from build123d import *

# Parameters (mm, degrees)
SKETCH_3_W          = 88.5
SKETCH_3_H          = 114.5
SKETCH_3_W_2        = 36.5
SKETCH_3_H_2        = 36.5
SKETCH_3_W_3        = 50.5
SKETCH_3_H_3        = 73.5
SKETCH_3_W_4        = 33.5
SKETCH_3_H_4        = 70.5
SKETCH_3_W_5        = 25.5
SKETCH_3_H_5        = 21.5
EXTRUDE_1_DEPTH     = 25
SKETCH_3_3_W        = 36.5
SKETCH_3_3_H        = 36.5
SKETCH_3_3_R        = 2.1
SKETCH_3_3_W_2      = 50.5
SKETCH_3_3_H_2      = 73.5
SKETCH_3_3_W_3      = 33.5
SKETCH_3_3_H_3      = 70.5
SKETCH_3_3_R_2      = 2.5
SKETCH_3_3_W_4      = 25.5
SKETCH_3_3_H_4      = 21.5
EXTRUDE_2_DEPTH     = 1.5
SKETCH_3_5_R        = 2.1
SKETCH_3_5_R_2      = 1.25
SKETCH_3_5_R_3      = 2.5
SKETCH_3_5_R_4      = 1.5
EXTRUDE_4_DEPTH     = 4.5
CUT_EXTRUDE_1_DEPTH = 17.5
CUT_EXTRUDE_2_REACH = 148.859
SKETCH_5_W          = 40
SKETCH_5_H          = 10
SKETCH_5_W_2        = 11
SKETCH_5_H_2        = 5


with BuildPart() as part:
    # 草图3 → 凸台-拉伸1 (new body)
    with BuildSketch(Plane(origin=(0, 0, 0), x_dir=(1, 0, 0), z_dir=(0, 1, 0))):
        with Locations((44.25, 57.25)):
            Rectangle(SKETCH_3_W, SKETCH_3_H)
        Polygon((39.5, 1.5), (39.5, 38), (53.5, 38), (53.5, 41), (87, 41), (87, 24.5), (60, 24.5), (60, 1.5), align=None, mode=Mode.SUBTRACT)
        with Locations((19.75, 19.75)):
            Rectangle(SKETCH_3_W_2, SKETCH_3_H_2, mode=Mode.SUBTRACT)
        with Locations((26.75, 76.25)):
            Rectangle(SKETCH_3_W_3, SKETCH_3_H_3, mode=Mode.SUBTRACT)
        with Locations((70.25, 77.75)):
            Rectangle(SKETCH_3_W_4, SKETCH_3_H_4, mode=Mode.SUBTRACT)
        with Locations((74.25, 12.25)):
            Rectangle(SKETCH_3_W_5, SKETCH_3_H_5, mode=Mode.SUBTRACT)
    extrude(amount=EXTRUDE_1_DEPTH)

    # 草图3<3> → 凸台-拉伸2 (add)
    # profile 1 of 5: a face of its own
    with BuildSketch(Plane(origin=(0, 0, 0), x_dir=(1, 0, 0), z_dir=(0, 1, 0))):
        Polygon((39.5, 38), (39.5, 1.5), (60, 1.5), (60, 24.5), (87, 24.5), (87, 41), (53.5, 41), (53.5, 38), align=None)
    # profile 2 of 5: a face of its own
    with BuildSketch(Plane(origin=(0, 0, 0), x_dir=(1, 0, 0), z_dir=(0, 1, 0))):
        with Locations((19.75, 19.75)):
            Rectangle(SKETCH_3_3_W, SKETCH_3_3_H)
        with Locations(Location((4, 35.5, 0), (0, 0, 270))):
            Circle(SKETCH_3_3_R, mode=Mode.SUBTRACT)
    # profile 3 of 5: a face of its own
    with BuildSketch(Plane(origin=(0, 0, 0), x_dir=(1, 0, 0), z_dir=(0, 1, 0))):
        with Locations((26.75, 76.25)):
            Rectangle(SKETCH_3_3_W_2, SKETCH_3_3_H_2)
        with Locations(Location((4.5, 42.5, 0), (0, 0, 270))):
            Circle(SKETCH_3_3_R, mode=Mode.SUBTRACT)
        with Locations(Location((49, 42.5, 0), (0, 0, 270))):
            Circle(SKETCH_3_3_R, mode=Mode.SUBTRACT)
        with Locations(Location((4.5, 109.8, 0), (0, 0, 270))):
            Circle(SKETCH_3_3_R, mode=Mode.SUBTRACT)
        with Locations(Location((49, 109.8, 0), (0, 0, 270))):
            Circle(SKETCH_3_3_R, mode=Mode.SUBTRACT)
    # profile 4 of 5: a face of its own
    with BuildSketch(Plane(origin=(0, 0, 0), x_dir=(1, 0, 0), z_dir=(0, 1, 0))):
        with Locations((70.25, 77.75)):
            Rectangle(SKETCH_3_3_W_3, SKETCH_3_3_H_3)
        with Locations(Location((56.5, 45.5, 0), (0, 0, 270))):
            Circle(SKETCH_3_3_R_2, mode=Mode.SUBTRACT)
        with Locations(Location((84, 110, 0), (0, 0, 270))):
            Circle(SKETCH_3_3_R_2, mode=Mode.SUBTRACT)
    # profile 5 of 5: a face of its own
    with BuildSketch(Plane(origin=(0, 0, 0), x_dir=(1, 0, 0), z_dir=(0, 1, 0))):
        with Locations((74.25, 12.25)):
            Rectangle(SKETCH_3_3_W_4, SKETCH_3_3_H_4)
        with Locations(Location((65, 13.9, 0), (0, 0, 270))):
            Circle(SKETCH_3_3_R_2, mode=Mode.SUBTRACT)
    extrude(amount=EXTRUDE_2_DEPTH)

    # 草图3<5> → 凸台-拉伸4 (add)
    # profile 1 of 8: a face of its own
    with BuildSketch(Plane(origin=(0, 0, 0), x_dir=(1, 0, 0), z_dir=(0, 1, 0))):
        with Locations(Location((4, 35.5, 0), (0, 0, 270))):
            Circle(SKETCH_3_5_R)
        with Locations(Location((4, 35.5, 0), (0, 0, 270))):
            Circle(SKETCH_3_5_R_2, mode=Mode.SUBTRACT)
    # profile 2 of 8: a face of its own
    with BuildSketch(Plane(origin=(0, 0, 0), x_dir=(1, 0, 0), z_dir=(0, 1, 0))):
        with Locations(Location((4.5, 42.5, 0), (0, 0, 270))):
            Circle(SKETCH_3_5_R)
        with Locations(Location((4.5, 42.5, 0), (0, 0, 270))):
            Circle(SKETCH_3_5_R_2, mode=Mode.SUBTRACT)
    # profile 3 of 8: a face of its own
    with BuildSketch(Plane(origin=(0, 0, 0), x_dir=(1, 0, 0), z_dir=(0, 1, 0))):
        with Locations(Location((49, 42.5, 0), (0, 0, 270))):
            Circle(SKETCH_3_5_R)
        with Locations(Location((49, 42.5, 0), (0, 0, 270))):
            Circle(SKETCH_3_5_R_2, mode=Mode.SUBTRACT)
    # profile 4 of 8: a face of its own
    with BuildSketch(Plane(origin=(0, 0, 0), x_dir=(1, 0, 0), z_dir=(0, 1, 0))):
        with Locations(Location((4.5, 109.8, 0), (0, 0, 270))):
            Circle(SKETCH_3_5_R)
        with Locations(Location((4.5, 109.8, 0), (0, 0, 270))):
            Circle(SKETCH_3_5_R_2, mode=Mode.SUBTRACT)
    # profile 5 of 8: a face of its own
    with BuildSketch(Plane(origin=(0, 0, 0), x_dir=(1, 0, 0), z_dir=(0, 1, 0))):
        with Locations(Location((49, 109.8, 0), (0, 0, 270))):
            Circle(SKETCH_3_5_R)
        with Locations(Location((49, 109.8, 0), (0, 0, 270))):
            Circle(SKETCH_3_5_R_2, mode=Mode.SUBTRACT)
    # profile 6 of 8: a face of its own
    with BuildSketch(Plane(origin=(0, 0, 0), x_dir=(1, 0, 0), z_dir=(0, 1, 0))):
        with Locations(Location((84, 110, 0), (0, 0, 270))):
            Circle(SKETCH_3_5_R_3)
        with Locations(Location((84, 110, 0), (0, 0, 270))):
            Circle(SKETCH_3_5_R_4, mode=Mode.SUBTRACT)
    # profile 7 of 8: a face of its own
    with BuildSketch(Plane(origin=(0, 0, 0), x_dir=(1, 0, 0), z_dir=(0, 1, 0))):
        with Locations(Location((56.5, 45.5, 0), (0, 0, 270))):
            Circle(SKETCH_3_5_R_3)
        with Locations(Location((56.5, 45.5, 0), (0, 0, 270))):
            Circle(SKETCH_3_5_R_4, mode=Mode.SUBTRACT)
    # profile 8 of 8: a face of its own
    with BuildSketch(Plane(origin=(0, 0, 0), x_dir=(1, 0, 0), z_dir=(0, 1, 0))):
        with Locations(Location((65, 13.9, 0), (0, 0, 270))):
            Circle(SKETCH_3_5_R_3)
        with Locations(Location((65, 13.9, 0), (0, 0, 270))):
            Circle(SKETCH_3_5_R_2, mode=Mode.SUBTRACT)
    extrude(amount=EXTRUDE_4_DEPTH)

    # 草图4 → 切除-拉伸1 (cut)
    with BuildSketch(Plane(origin=(0, 25, 0), x_dir=(1, 0, 0), z_dir=(0, 1, 0))):
        Polygon((61.5, 1.5), (38, 1.5), (38, 38), (61.5, 38), (61.5, 44.990704611), (82.058079057, 44.990704611), (82.058079057, 21.502306723), (61.5, 21.502306723), align=None)
    extrude(amount=-CUT_EXTRUDE_1_DEPTH, mode=Mode.SUBTRACT)

    # 草图5 → 切除-拉伸2 (cut, up to next)
    with BuildSketch(Plane.ZY, mode=Mode.PRIVATE) as cut_extrude_2_sk1:
        with Locations((-64.5, 11.5)):
            Rectangle(SKETCH_5_W, SKETCH_5_H)
    cut_extrude_2_tool1 = extrude(cut_extrude_2_sk1.sketch, amount=-CUT_EXTRUDE_2_REACH, mode=Mode.PRIVATE) & part.part
    # 草图5 → 切除-拉伸2 (cut, up to next)
    with BuildSketch(Plane.ZY, mode=Mode.PRIVATE) as cut_extrude_2_sk2:
        with Locations((-9, 9)):
            Rectangle(SKETCH_5_W_2, SKETCH_5_H_2)
    cut_extrude_2_tool2 = extrude(cut_extrude_2_sk2.sketch, amount=-CUT_EXTRUDE_2_REACH, mode=Mode.PRIVATE) & part.part
    add(cut_extrude_2_tool1.solids().sort_by_distance((0, 11.5, -64.5))[0], mode=Mode.SUBTRACT)
    add(cut_extrude_2_tool2.solids().sort_by_distance((0, 9, -9))[0], mode=Mode.SUBTRACT)


solid = part.part
Verification items for the finished model (mm, model axes). A direction names the side the tool comes from. Give positions to 0.01 mm unless a question says otherwise; leave off trailing zeros. Write each loop counter-clockwise with the first axis right and the second up, starting at its lowest first coordinate (ties: lowest second). Pieces come first, ordered by that corner, then holes.
(1) Cross-section at C-C (y = 23.25). Enter the section's corners in (x, z), plus the area to 3 significant figures.
(2) Cross-section at D-D (x = 24). Enter the section's corners in (y, z).
(3) Gauge pin test, flat ends, axial feed: pin 1 (2.5 mm diameter, centred on x = 83, z = -109.5, fed in from +Y); pin 2 (6 mm diameter, centred on x = 34.5, z = -49, fed in from +Y); pin 3 (0.8 mm diameter, centred on x = 73.5, z = -42, fed in from +Y). Record the tip position at first contact, or that the pin passes through.
(4) Material ranges on line 1 (Z direction, x = 25, y = 3.5); line 2 (X direction, y = 17, z = -92); line 3 (Z direction, x = 82.5, y = 17), recorded low to high.
(5) Cross-section at B-B (z = -35.5). Enter the section's corners in (x, y), plus the area to 3 significant figures.
(6) Access from +Z, -Z, +X, -X, +Y, -Y to the whole of each face (thin tool, end or side, straight path). Record for faces 1 (the face through (50.24, 2.22, -42.66)), 2 (the face through (1.5, 18, -76)).
(7) Cross-section at A-A (x = 56.5). Enter the section's corners in (y, z).
Worked out:
1. outline: (0, -114.5) - (88.5, -114.5) - (88.5, 0) - (0, 0) - close; hole (1.5, -113) - (52, -113) - (52, -39.5) - (1.5, -39.5) - close; hole (1.5, -38) - (53.5, -38) - (53.5, -41) - (61.5, -41) - (61.5, -42.5) - (53.5, -42.5) - (53.5, -113) - (87, -113) - (87, -42.5) - (82.06, -42.5) - (82.06, -41) - (87, -41) - (87, -24.5) - (82.06, -24.5) - (82.06, -23) - (87, -23) - (87, -1.5) - (1.5, -1.5) - close
1. area: 815 mm2
2. outline: (0, -114.5) - (25, -114.5) - (25, -113) - (1.5, -113) - (1.5, -39.5) - (25, -39.5) - (25, -38) - (1.5, -38) - (1.5, -1.5) - (25, -1.5) - (25, 0) - (0, 0) - close
3. pin 1: stops at y = 4.5
3. pin 2: stops at y = 1.5
3. pin 3: stops at y = 7.5
4. line 1: z = -114.5 to -113, -39.5 to -38, -1.5 to 0
4. line 2: x = 0 to 1.5, 52 to 53.5, 87 to 88.5
4. line 3: z = -114.5 to -113, -42.5 to -41, -24.5 to -23, -1.5 to 0
5. outline: (0, 0) - (2.75, 0) - (2.75, 4.5) - (1.9, 4.5) - (1.9, 1.5) - (1.5, 1.5) - (1.5, 25) - (0, 25) - close; (5.25, 0) - (88.5, 0) - (88.5, 25) - (87, 25) - (87, 1.5) - (39.5, 1.5) - (39.5, 7.5) - (38, 7.5) - (38, 1.5) - (6.1, 1.5) - (6.1, 4.5) - (5.25, 4.5) - close
5. area: 214 mm2
6. face 1: +Y, -Y
6. face 2: +Y
7. outline: (0, -114.5) - (25, -114.5) - (25, -113) - (1.5, -113) - (1.5, -48) - (4.5, -48) - (4.5, -47) - (0, -47) - close; (0, -44) - (4.5, -44) - (4.5, -43) - (1.5, -43) - (1.5, -42.5) - (25, -42.5) - (25, -41) - (1.5, -41) - (1.5, -1.5) - (25, -1.5) - (25, 0) - (0, 0) - close
